Source: three-view drawing plus pictorial views. Frame: mm from the lowest corner of the part. A direction names the side the tool comes from. Round coordinates to 2 decimals unless told otherwise and drop trailing zeros. Loops run counter-clockwise (first coordinate to the right, second up) from the corner with the lowest first, then second, coordinate; pieces in that order, holes last. Notation, with made-up numbers: M 25,89 L 76,89 A28 ccw 76,122 Z; hole C -3,68 d11. An arc over 180 degrees is marked long. Answer as a JSON object with one key per item and string values.
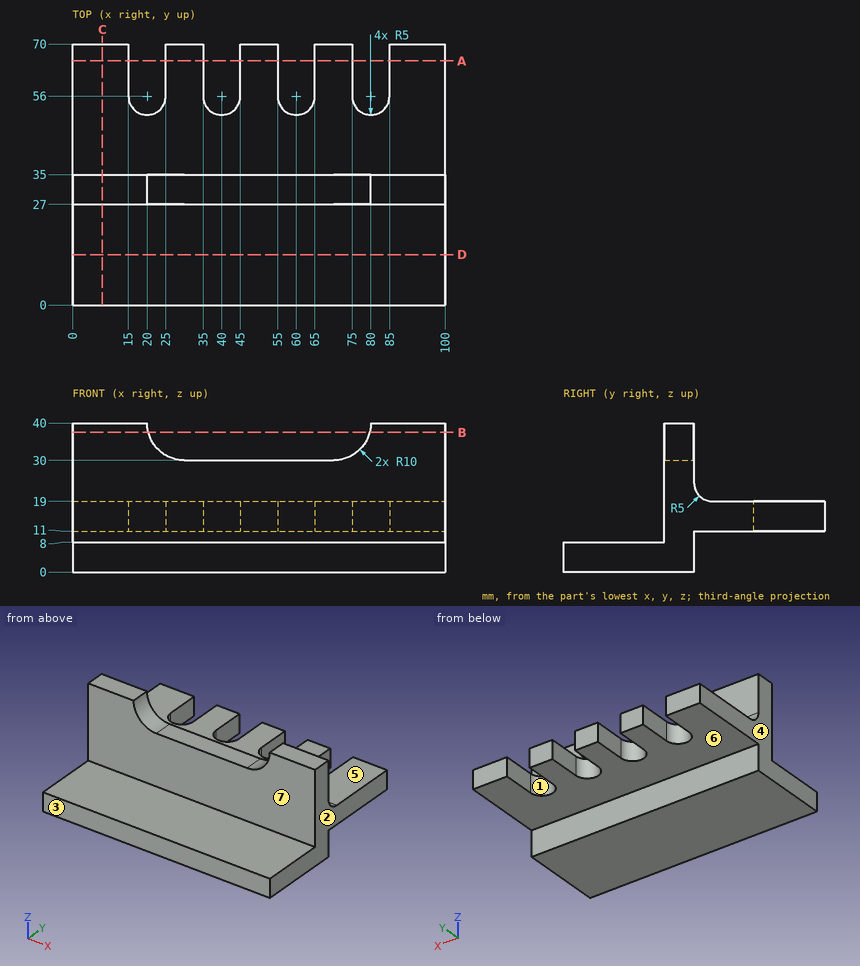
1) Line query: probe 1 along Z at (x, y) = (66.5, 58.5); probe 2 along Z at (x, y) = (93.5, 37); probe 3 along Y at (x, z) = (94, 2). Output: solid intervals per line, ascending.
Geometry results:
{"probe 1": "11 to 19", "probe 2": "11 to 20", "probe 3": "0 to 35"}
2) Cut plane B-B on z = 37.5. Return the cut outline in (x, y), and give its area (3 significant figures).
Geometry results:
{"outline": "M 0,27 L 20.32,27 L 20.32,35 L 0,35 Z; M 79.68,27 L 100,27 L 100,35 L 79.68,35 Z", "area": "325 mm2"}
3) Set-up query: the marked faces 5, 6 and 7. Return all of +Z, -Z, +X, -X, +Y, -Y with unobstructed straight access to the full face (end or side cutting, diameter ignored); none if empty.
Geometry results:
{"face 5": "+Z, +X, -X, +Y", "face 6": "-Z, +X, -X, +Y", "face 7": "+Z, +X, -X, -Y"}
4) Cut plane C-C on x = 8. Return the cut outline in (y, z).
Geometry results:
{"outline": "M 0,0 L 35,0 L 35,11 L 70,11 L 70,19 L 40,19 A5 cw 35,24 L 35,40 L 27,40 L 27,8 L 0,8 Z"}
5) Cut plane D-D on y = 13.5. Return the cut outline in (x, z), and give its area (3 significant figures).
Geometry results:
{"outline": "M 0,0 L 100,0 L 100,8 L 0,8 Z", "area": "800 mm2"}
6) Cut plane A-A on y = 65.5. Return the cut outline in (x, z), and give its area (3 significant figures).
Geometry results:
{"outline": "M 0,11 L 15,11 L 15,19 L 0,19 Z; M 25,11 L 35,11 L 35,19 L 25,19 Z; M 45,11 L 55,11 L 55,19 L 45,19 Z; M 65,11 L 75,11 L 75,19 L 65,19 Z; M 85,11 L 100,11 L 100,19 L 85,19 Z", "area": "480 mm2"}
7) Pull-direction query (X, two-part tool) for the marked faces 1, 2, 3 and 4; classes: +X half, -X half, draft (parallel to the pull), parting line (faces both ways), or undercut.
Geometry results:
{"face 1": "undercut", "face 2": "+X half", "face 3": "draft", "face 4": "-X half"}
8) First-contact query: pin 1 (4 mm diameter, centred on x = 10.5, z = 28, fed in from -Y); pin 2 (6.5 mm diameter, centred on x = 56.5, y = 32.5, fed in from +Z); pin 3 (5.5 mm diameter, centred on x = 46, z = 7, fed in from +Y). Flat tips, straight axial feed; report the tip coordinate or a pass-through.
Geometry results:
{"pin 1": "y = 27", "pin 2": "z = 30", "pin 3": "y = 35"}
